Here's how the part is built. I have some questions about the finished solid (model axes, mm). A direction names the side the tool comes from. Coordinates: 2 decimals unless noted, no trailing zeros. Order: outer loops, then holes, each group sorted by start corner. A loop starts at its lowest first (then second) coordinate and runs counter-clockwise, first axis right, second up. Notation, with made-up numbers: M 52,53 L 81,53 A18 cw 81,79 Z; hole C 75.5,6.5 d4. An arc over 180 degrees is marked long. Answer as CSV lines item,"result". Start each with the question number.
```python
from build123d import *

# Parameters (mm, degrees)
BOSS_EXTRUDE1_DEPTH   = 10
BOSS_EXTRUDE2_DEPTH   = 10
F_6_CLEARANCE_HOLE1_D = 3.7973
F_6_CLEARANCE_HOLE2_D = 3.7973
FILLET1_R             = 5


with BuildPart() as part:
    # Sketch1 → Boss-Extrude1 (new body)
    with BuildSketch(Plane(origin=(0, 0, 0), x_dir=(1, 0, 0), z_dir=(0, 1, 0))):
        with BuildLine():
            Line((-1.25, 14.477642868), (-1.25, 5.868347297))
            ThreePointArc((-1.25, 5.868347297), (0, -6), (1.25, 5.868347297))
            Line((1.25, 5.868347297), (1.25, 14.477642868))
            Line((1.25, 14.477642868), (2.75, 14.477642868))
            Line((2.75, 14.477642868), (2.75, 6.977642868))
            ThreePointArc((2.75, 6.977642868), (0, -7.5), (-2.75, 6.977642868))
            Line((-2.75, 6.977642868), (-2.75, 14.477642868))
            Line((-2.75, 14.477642868), (-1.25, 14.477642868))
        make_face()
    extrude(amount=BOSS_EXTRUDE1_DEPTH)

    # Loft1: read off the stored shape, not the designer's step
    # Loft1: loft between two sections, ruled curve by curve
    loft1_from = [
        Edge.make_bspline([(1.25, 10, -5.868347297), (10.900494926, 10, -3.812722767), (9.866997746, 10, 6), (-9.866997746, 10, 6), (-10.900494926, 10, -3.812722767), (-1.25, 10, -5.868347297)], [0, 0, 0, 0, 0.5, 0.5, 1, 1, 1, 1], 3, [1, 0.162539502, 0.065529731, 0.065529731, 0.162539502, 1]),
        Edge.make_bspline([(-1.25, 10, -7.395099729), (-13.876567029, 10, -5.260820359), (-12.805676217, 10, 7.5), (12.805676217, 10, 7.5), (13.876567029, 10, -5.260820359), (1.25, 10, -7.395099729)], [0, 0, 0, 0, 0.5, 0.5, 1, 1, 1, 1], 3, [1, 0.151386494, 0.058902089, 0.058902089, 0.151386494, 1]),
        Edge.make_line((-1.25, 10, -7.395099729), (-1.25, 10, -5.868347297)),
        Edge.make_line((1.25, 10, -5.868347297), (1.25, 10, -7.395099729)),
    ]
    loft1_to = [
        Edge.make_bspline([(3, 12.5, -3.010398645), (6.15488313, 12.5, 0.133586757), (4.453979318, 12.5, 4.25), (-4.453979318, 12.5, 4.25), (-6.15488313, 12.5, 0.133586757), (-3, 12.5, -3.010398645)], [0, 0, 0, 0, 0.5, 0.5, 1, 1, 1, 1], 3, [1, 0.345653128, 0.203217328, 0.203217328, 0.345653128, 1]),
        Edge.make_bspline([(-3, 12.5, -4.905354218), (-9.124128689, 12.5, -1.159980234), (-7.178633469, 12.5, 5.75), (7.178633469, 12.5, 5.75), (9.124128689, 12.5, -1.159980234), (3, 12.5, -4.905354218)], [0, 0, 0, 0, 0.5, 0.5, 1, 1, 1, 1], 3, [1, 0.264204167, 0.135803041, 0.135803041, 0.264204167, 1]),
        Edge.make_line((-3, 12.5, -4.905354218), (-3, 12.5, -3.010398645)),
        Edge.make_line((3, 12.5, -3.010398645), (3, 12.5, -4.905354218)),
    ]
    loft1 = Solid(Shell([*[Face.make_surface_from_curves(loft1_from[k], loft1_to[k]) for k in range(4)], Face(Wire(loft1_from)), Face(Wire(loft1_to))]))
    add(loft1)

    # Sketch4 → Boss-Extrude2 (add)
    with BuildSketch(Plane(origin=(0, 12.5, 0), x_dir=(1, 0, 0), z_dir=(0, 1, 0))):
        with BuildLine():
            Line((-1.75, 5.123626074), (-1.75, 12.206169214))
            Line((-1.75, 12.206169214), (-3.25, 12.206169214))
            Line((-3.25, 12.206169214), (-3.25, 4.74341649))
            ThreePointArc((-3.25, 4.74341649), (0, -5.75), (3.25, 4.74341649))
            Line((3.25, 4.74341649), (3.25, 12.206169214))
            Line((3.25, 12.206169214), (1.75, 12.206169214))
            Line((1.75, 12.206169214), (1.75, 5.123626074))
            Line((1.75, 5.123626074), (1.75, 3.596873642))
            ThreePointArc((1.75, 3.596873642), (0, -4), (-1.75, 3.596873642))
            Line((-1.75, 3.596873642), (-1.75, 5.123626074))
        make_face()
    extrude(amount=BOSS_EXTRUDE2_DEPTH)

    # #6 Clearance Hole1 (through all)
    with Locations(Plane.ZY.offset(2.75)):
        with Locations((-10.727642082, 5)):
            Hole(F_6_CLEARANCE_HOLE1_D / 2)

    # #6 Clearance Hole2 (through all)
    with Locations(Plane.ZY.offset(3.25)):
        with Locations((-8.474792852, 17.5)):
            Hole(F_6_CLEARANCE_HOLE2_D / 2)

    # Fillet1
    fillet1_edges = [part.edges().sort_by_distance(p)[0] for p in [
        (2, 0, -14.477642868),
        (-2, 0, -14.477642868),
        (-2.5, 12.5, -12.206169214),
        (2.5, 12.5, -12.206169214),
        (-2.5, 22.5, -12.206169214),
        (2.5, 22.5, -12.206169214),
        (2, 10, -14.477642868),
        (-2, 10, -14.477642868),
    ]]
    fillet(fillet1_edges, radius=FILLET1_R - 0.0001)  # a hair under: the kernel refuses the full size


solid = part.part
```
1) I need wall thicknesses on line 1 (X direction, y = 8.25, z = -7.5); line 2 (Z direction, x = -2, y = 18.25); line 3 (X direction, y = 7, z = 0). Which ranges of each line are inside material? Lowest first, please. Write a range as [from, to].
2) Which directions (+Z, -Z, +X, -X, +Y, -Y) give clear straight access to the entire face, cutting with the end or side of a thin tool? Please do faces 5 (the face through (-1.75, 19, -7)), 6 (the face through (-2.75, 3.8, -9)), 7 (the face through (-2.51, 14.004, -10.78)).
3) Suppose I cut it at A-A on y = 16.5. Please give me the cut outline in (x, z), plus the area to 3 significant figures.
4) Suppose I cut it at C-C on y = 8. Please give me the cut outline in (x, z).
5) If we mould it in two halves opening along Z, with no side actions, what happens to faces 1 (the face through (2, 10, -8)), 2 (the face through (0.29, 4.93, 7.494)), 3 (the face through (2, 12.5, -4)), 4 (the face through (2.49, 21.074, -10.703))? For each: released by +Z, released by -Z, zero draft, split by the parting line, or undercut.
6) Will these pins go through, and if not, where does the flat tip stop? pin 1 Ø4.5 at (x, z) = (0, 0) entering from -Y; pin 2 Ø6 at (x, y) = (-1.5, 7) entering from +Z; pin 3 Ø8 at (y, z) = (7.5, -12) entering from -X; pin 4 Ø1 at (x, y) = (-4.5, 3) entering from -Z.
7) Suppose I cut it at B-B on y = 20.5. Please give me the cut outline in (x, z).
Output:
1,line 1,"[-2.75, -1.25], [1.25, 2.75]"
1,line 2,"[-12.15, -10.22], [-6.73, -3.46], [3.46, 5.39]"
1,line 3,"[-7.5, -6], [6, 7.5]"
2,face 5,"-Z, +Y"
2,face 6,"-Z, -X, -Y"
2,face 7,"-Z, +X, -X"
3,outline,"M -3.25,-12.11 L -1.75,-12.11 L -1.75,-10.09 L -3.25,-10.09 Z; M -3.25,-6.86 L -1.75,-6.86 L -1.75,-3.6 A4 cw long 1.75,-3.6 L 1.75,-6.86 L 3.25,-6.86 L 3.25,-4.74 A5.75 ccw long -3.25,-4.74 Z; M 1.75,-12.11 L 3.25,-12.11 L 3.25,-10.09 L 1.75,-10.09 Z"
3,area,"58.5 mm²"
4,outline,"M -2.75,-13.48 L -1.25,-13.48 L -1.25,-5.87 A6 cw long 1.25,-5.87 L 1.25,-13.48 L 2.75,-13.48 L 2.75,-6.98 A7.5 ccw long -2.75,-6.98 Z"
5,face 1,"zero draft"
5,face 2,"split by the parting line"
5,face 3,"undercut"
5,face 4,"released by -Z"
6,pin 1,"through"
6,pin 2,"z = 7.5"
6,pin 3,"x = -2.75"
6,pin 4,"z = -6.34"
7,outline,"M -3.25,-11.21 L -1.75,-11.21 L -1.75,-3.6 A4 cw long 1.75,-3.6 L 1.75,-11.21 L 3.25,-11.21 L 3.25,-4.74 A5.75 ccw long -3.25,-4.74 Z"
